The listing builds one solid part. Answer for the finished solid, in the listing's coordinates (mm). A direction names the side the tool comes from. Round coordinates to 2 decimals unless told otherwise and drop trailing zeros. Write each loop counter-clockwise with the first axis right and the second up, starting at its lowest first coordinate (ties: lowest second). Pieces come first, ordered by that corner, then holes. Notation, with made-up numbers: (10, 2.25) - (16, 2.25) arc R32 ccw to (16, 36.25) - close; hole circle Ø11 at (3.5, 26.25). An arc over 180 degrees is marked (long way). Answer as CSV lines item,"result". Start each with the question number.
Item 1: A cutting plane is placed at A-A on y = 7. Determine the outline of the cut face in (x, z), and give its area (3 significant figures).
Item 2: Straight lines are drawn through the part: line 1 along X through (y, z) = (-23.9, -8.7); line 2 along Z through (x, y) = (-21, -10); line 3 along Y through (x, z) = (-5, -13). For each, find the intervals that lie inside material, in ascending order. Write a range as [from, to].
Item 3: Flat-ended cylindrical pins translate along their axes: pin 1 (0.8 mm diameter, centred on x = 10, z = -0.5, fed in from +Y); pin 2 (1.4 mm diameter, centred on y = -23, z = -5, fed in from -X); pin 3 (0.8 mm diameter, centred on y = -23.5, z = -10, fed in from +X). Find the tip coordinate at first contact, or state that the pin passes through.
Item 4: A cutting plane is placed at B-B on x = -6. Determine the outline of the cut face in (y, z).
Item 5: For a pull along X with two mould halves and no side action, classify faces 1 (the cylindrical face through (26.748, -23.855, -14.987)), 2 (the cylindrical face through (-21.102, 21.787, -0.355)), 3 (the flat face through (0, -24.2, -9)), 4 (the cylindrical face through (-25.14, 19.15, -0.35)) as pulls with the +X half, pulls with the -X half, needs draft (parallel to the pull), parting line crosses it, or undercut.
Item 6: Which of the six approach directions +Z, -Z, +X, -X, +Y, -Y give full straight-line access (tool end or side, diameter ignored) to faces 5 (the cylindrical face through (25.07, -14.15, -0.35)), 6 (the flat face through (0, -20, -0.7)), 7 (the cylindrical face through (18.61, -23.85, -9.59))?
```python
from build123d import *

# Parameters (mm, degrees)
BASE_FLANGE1_DEPTH    = 0.7
EDGE_FLANGE1_DEPTH    = 55
CUT_EXTRUDE1_DEPTH    = 10
CUT_EXTRUDE2_REACH    = 59.839
SKETCH9_R             = 1.65
BREAK_CORNER1_START   = -24.2
BREAK_CORNER1_DEPTH   = 0.7
BREAK_CORNER1_START_2 = -0.7
BREAK_CORNER1_2_DEPTH = 0.7


# Read off the part's stored shape, not the designer's step: Break-Corner1
# Sheet-metal steps are written as plain solids
with BuildPart() as part:
    # Sketch2 → Base-Flange1 (new body)
    with BuildSketch(Plane.XY):
        Polygon((20.35, 22.5), (31.35, 22.5), (31.35, -22.5), (-31.35, -22.5), (-31.35, 22.5), (-20.35, 22.5), (-20.35, -17.5), (20.35, -17.5), align=None)
    extrude(amount=-BASE_FLANGE1_DEPTH)

    # Edge-Flange1 section (across the edge) → Edge-Flange1 (add)
    with BuildSketch(Plane(origin=(27.5, -23.5, -0.7), x_dir=(0, 1, 0), z_dir=(-1, 0, 0))):
        with BuildLine():
            Line((-0.7, 1), (-0.7, 15))
            Line((-0.7, 15), (0, 15))
            Line((0, 15), (0, 1))
            ThreePointArc((0, 1), (0.292893219, 0.292893219), (1, 0))
            Line((1, 0), (1, -0.7))
            ThreePointArc((1, -0.7), (-0.202081528, -0.202081528), (-0.7, 1))
        make_face()
    extrude(amount=EDGE_FLANGE1_DEPTH)

    # Sketch8 → Cut-Extrude1 (cut)
    with BuildSketch(Plane.XY):
        with BuildLine():
            Line((-23.458, 17.5), (-23.458, -12.5))
            ThreePointArc((-23.458, -12.5), (-25.108, -14.15), (-26.758, -12.5))
            Line((-26.758, -12.5), (-26.758, 17.5))
            ThreePointArc((-26.758, 17.5), (-25.108, 19.15), (-23.458, 17.5))
        make_face()
        with BuildLine():
            Line((23.458, 17.5), (23.458, -12.5))
            ThreePointArc((23.458, -12.5), (25.108, -14.15), (26.758, -12.5))
            Line((26.758, -12.5), (26.758, 17.5))
            ThreePointArc((26.758, 17.5), (25.108, 19.15), (23.458, 17.5))
        make_face()
    extrude(amount=-CUT_EXTRUDE1_DEPTH, mode=Mode.SUBTRACT)

    # Sketch9 → Cut-Extrude2 (cut, up to next)
    with BuildSketch(Plane(origin=(0, -23.5, 0), x_dir=(1, 0, 0), z_dir=(0, 1, 0)), mode=Mode.PRIVATE) as cut_extrude2_sk1:
        with Locations(Location((-20, 8.7, 0), (0, 0, 270))):
            Circle(SKETCH9_R)
    cut_extrude2_tool1 = extrude(cut_extrude2_sk1.sketch, amount=-CUT_EXTRUDE2_REACH, mode=Mode.PRIVATE) & part.part
    # Sketch9 → Cut-Extrude2 (cut, up to next)
    with BuildSketch(Plane(origin=(0, -23.5, 0), x_dir=(1, 0, 0), z_dir=(0, 1, 0)), mode=Mode.PRIVATE) as cut_extrude2_sk2:
        with Locations(Location((20, 8.7, 0), (0, 0, 90))):
            Circle(SKETCH9_R)
    cut_extrude2_tool2 = extrude(cut_extrude2_sk2.sketch, amount=-CUT_EXTRUDE2_REACH, mode=Mode.PRIVATE) & part.part
    add(cut_extrude2_tool1.solids().sort_by_distance((-20, -23.5, -8.7))[0], mode=Mode.SUBTRACT)
    add(cut_extrude2_tool2.solids().sort_by_distance((20, -23.5, -8.7))[0], mode=Mode.SUBTRACT)

    # Break-Corner1 outline → Break-Corner1 (cut)
    with BuildSketch(Plane(origin=(0, 0, 0), x_dir=(1, 0, 0), z_dir=(0, 1, 0)).offset(BREAK_CORNER1_START)):
        with BuildLine():
            Line((27.5, 15.7), (25, 15.7))
            ThreePointArc((25, 15.7), (26.767766953, 14.967766953), (27.5, 13.2))
            Line((27.5, 13.2), (27.5, 15.7))
        make_face()
        with BuildLine():
            ThreePointArc((-27.5, 13.2), (-26.767766953, 14.967766953), (-25, 15.7))
            Line((-25, 15.7), (-27.5, 15.7))
            Line((-27.5, 15.7), (-27.5, 13.2))
        make_face()
    extrude(amount=BREAK_CORNER1_DEPTH, mode=Mode.SUBTRACT)

    # Break-Corner1 2 outline → Break-Corner1 2 (cut)
    with BuildSketch(Plane.XY.offset(BREAK_CORNER1_START_2)):
        with BuildLine():
            ThreePointArc((20.35, 20), (21.082233047, 21.767766953), (22.85, 22.5))
            Line((22.85, 22.5), (20.35, 22.5))
            Line((20.35, 22.5), (20.35, 20))
        make_face()
        with BuildLine():
            ThreePointArc((28.85, 22.5), (30.617766953, 21.767766953), (31.35, 20))
            Line((31.35, 20), (31.35, 22.5))
            Line((31.35, 22.5), (28.85, 22.5))
        make_face()
        with BuildLine():
            ThreePointArc((31.35, -20), (30.617766953, -21.767766953), (28.85, -22.5))
            Line((28.85, -22.5), (31.35, -22.5))
            Line((31.35, -22.5), (31.35, -20))
        make_face()
        with BuildLine():
            Line((-20.35, 22.5), (-22.85, 22.5))
            ThreePointArc((-22.85, 22.5), (-21.082233047, 21.767766953), (-20.35, 20))
            Line((-20.35, 20), (-20.35, 22.5))
        make_face()
        with BuildLine():
            Line((-31.35, 22.5), (-31.35, 20))
            ThreePointArc((-31.35, 20), (-30.617766953, 21.767766953), (-28.85, 22.5))
            Line((-28.85, 22.5), (-31.35, 22.5))
        make_face()
        with BuildLine():
            ThreePointArc((-28.85, -22.5), (-30.617766953, -21.767766953), (-31.35, -20))
            Line((-31.35, -20), (-31.35, -22.5))
            Line((-31.35, -22.5), (-28.85, -22.5))
        make_face()
    extrude(amount=BREAK_CORNER1_2_DEPTH, mode=Mode.SUBTRACT)


solid = part.part
```
Geometry says:
1,outline,"(-31.35, -0.7) - (-26.76, -0.7) - (-26.76, 0) - (-31.35, 0) - close; (-23.46, -0.7) - (-20.35, -0.7) - (-20.35, 0) - (-23.46, 0) - close; (20.35, -0.7) - (23.46, -0.7) - (23.46, 0) - (20.35, 0) - close; (26.76, -0.7) - (31.35, -0.7) - (31.35, 0) - (26.76, 0) - close"
1,area,"10.8 mm^2"
2,line 1,"x = [-27.5, -21.65], [-18.35, 18.35], [21.65, 27.5]"
2,line 2,"z = [-0.7, 0]"
2,line 3,"y = [-24.2, -23.5]"
3,pin 1,"stops at y = -17.5"
3,pin 2,"stops at x = -27.5"
3,pin 3,"stops at x = 27.5"
4,outline,"(-24.2, -15.7) - (-23.5, -15.7) - (-23.5, -1.7) arc R1 cw to (-22.5, -0.7) - (-17.5, -0.7) - (-17.5, 0) - (-22.5, 0) arc R1.7 ccw to (-24.2, -1.7) - close"
5,face 1,"pulls with the +X half"
5,face 2,"undercut"
5,face 3,"needs draft"
5,face 4,"undercut"
6,face 5,"+Z, -Z"
6,face 6,"-Z, +X, -X, +Y"
6,face 7,"+Y, -Y"
